```python
from build123d import *

# Parameters (mm, degrees)
F0_R     = 12
F1_DEPTH = 2.032
F2_SIZE  = 0.762
F3_R     = 2.4
F4_DEPTH = 1.6
F4_TAPER = -4


with BuildPart() as f1:
    # F0 (on Top) → F1 (new body)
    with BuildSketch(Plane.XY):
        Circle(F0_R)
    extrude(amount=F1_DEPTH)

    # F2
    f2_edges = [f1.edges().sort_by_distance(p)[0] for p in [
        (-12, 0, 2.032),
    ]]
    chamfer(f2_edges, length=F2_SIZE)

    # F3 (on face) → F4 (join)
    with BuildSketch(Plane.XY.offset(2.032)):
        with Locations((4, 0)):
            Circle(F3_R)
        with Locations((-4, 0)):
            Circle(F3_R)
    extrude(amount=F4_DEPTH, taper=F4_TAPER)


solid = f1.part
```
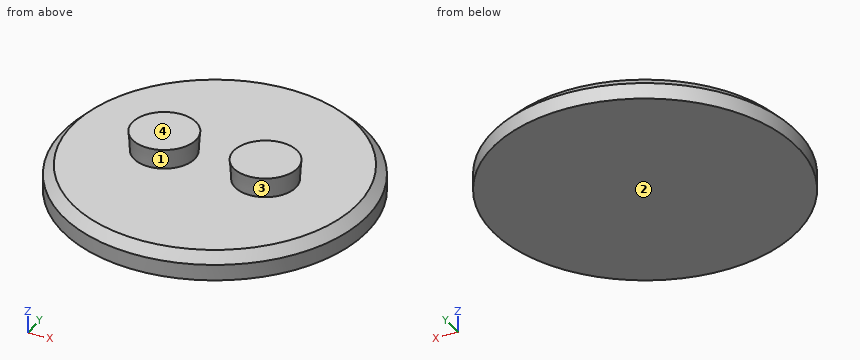
Could you check a few things on this model? Use its own coordinates, in mm. Face numbers are marked on the shaded views. A direction names the side the tool comes from. Coordinates: 2 decimals unless noted, no trailing zeros. Write each loop counter-clockwise with the first axis right and the second up, starting at its lowest first coordinate (ties: lowest second). Pieces come first, ordered by that corner, then holes. Notation, with made-up numbers: (4, 68) -> (34, 68) arc R16 ccw to (34, 80) -> close; hole circle Ø10 at (33.25, 34.5). An arc over 180 degrees is marked (long way). Write item = value, one per line. Start each with the question number.
(1) I need wall thicknesses on line 1 (Z direction, x = 8.75, y = -3); line 2 (X direction, y = 2, z = 2.5); line 3 (Y direction, x = -4.25, z = 2.1). Which ranges of each line are inside material? Lowest first, please. Write a range as [from, to].
(2) Will these pins go through, and if not, where does the flat tip stop? pin 1 (1 mm diameter, centred on x = 1.5, y = 2, fed in from +Z); pin 2 (5 mm diameter, centred on x = 6, y = 1.5, fed in from -Z).
(3) Which directions (+Z, -Z, +X, -X, +Y, -Y) give clear straight access to the entire face, cutting with the end or side of a thin tool? Please do the marked faces 1 and 2.
(4) I want a section at B-B (z = 1.6). Please give me the cut outline in (x, y).
(5) We'd pull the mould along X, two halves only. Please class the marked faces 3 and 4: released by +X, released by -X, zero draft, split by the parting line, or undercut.
(6) I want a section at A-A (x = 0). Please give me the cut outline in (y, z), plus the area to 3 significant figures.
Result set:
q1.line_1 = [0, 2.03]
q1.line_2 = [-5.38, -2.62], [2.62, 5.38]
q1.line_3 = [-2.39, 2.39]
q2.pin_1 = 2.03
q2.pin_2 = 0
q3.face_1 = none
q3.face_2 = -Z, +X, -X, +Y, -Y
q4.outline = circle Ø23.34 at (0, 0)
q5.face_3 = undercut
q5.face_4 = zero draft
q6.outline = (-12, 0) -> (12, 0) -> (12, 1.27) -> (11.24, 2.03) -> (-11.24, 2.03) -> (-12, 1.27) -> close
q6.area = 48.2 mm2
